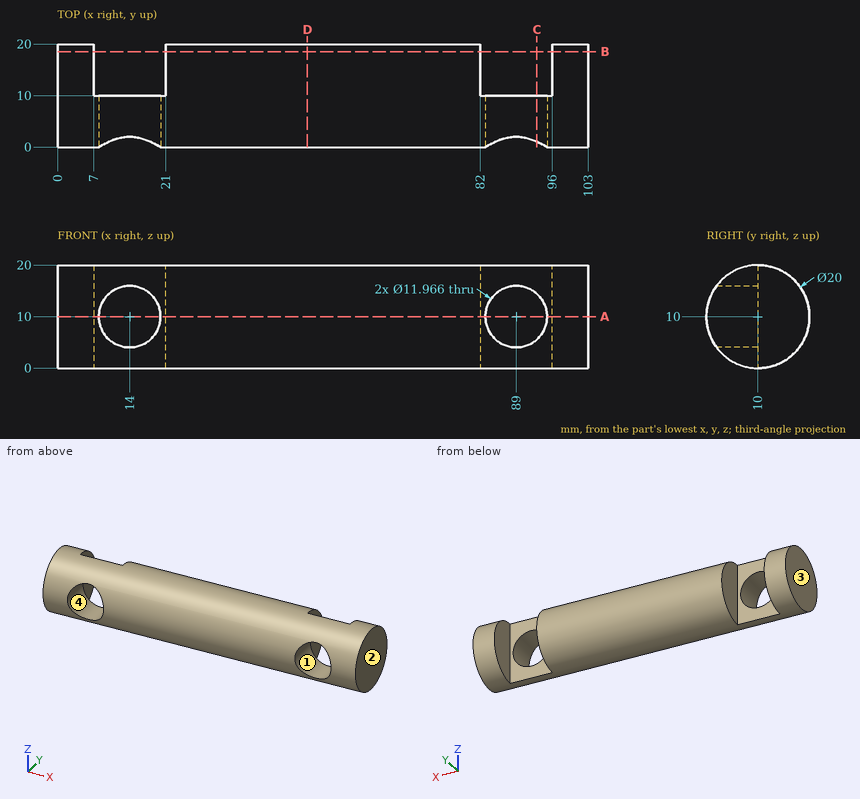
Geometry: see drawing. Coordinates: mm, zero at the bounding-box minimum. Round coordinates to 2 decimals unless told otherwise and drop trailing zeros. Loops run counter-clockwise (first coordinate to the right, second up) from the corner with the lowest first, then second, coordinate; pieces in that order, holes last.
(1) Section query A-A (z = 10). Output: boundary loops of the cut face in (x, y).
From the geometry:
outline: (0, 0) - (8.02, 0) - (8.02, 10) - (7, 10) - (7, 20) - (0, 20) - close; (19.98, 0) - (83.02, 0) - (83.02, 10) - (82, 10) - (82, 20) - (21, 20) - (21, 10) - (19.98, 10) - close; (94.98, 0) - (103, 0) - (103, 20) - (96, 20) - (96, 10) - (94.98, 10) - close
(2) Material intervals for probe 1 along X at (y, z) = (2.75, 10); probe 2 along X at (y, z) = (10.75, 17.5); probe 3 along Z at (x, y) = (72, 9.5), sorted ascending.
From the geometry:
probe 1: x = 0 to 8.02, 19.98 to 83.02, 94.98 to 103
probe 2: x = 0 to 7, 21 to 82, 96 to 103
probe 3: z = 0.01 to 19.99
(3) Section query C-C (x = 93). Output: boundary loops of the cut face in (y, z).
From the geometry:
outline: (1.04, 5.55) arc R10 ccw to (10, 0) - (10, 5.55) - close; (1.04, 14.45) - (10, 14.45) - (10, 20) arc R10 ccw to start
(4) Section query D-D (x = 48.5). Output: boundary loops of the cut face in (y, z), and give its area (3 significant figures).
From the geometry:
outline: circle Ø20 at (10, 10)
area: 314 mm2
(5) Contact query for flat-ended pins moving along their axis: pin 1 Ø10 at (x, y) = (56, 16) entering from +Z; pin 2 Ø3 at (x, z) = (84, 12) entering from -Y; pin 3 Ø3 at (x, z) = (46, 4.5) entering from +Y; pin 4 Ø11 at (x, z) = (14, 10) entering from -Y. Output: stop coordinate, or through.
From the geometry:
pin 1: stops at z = 19.95
pin 2: stops at y = 0.03
pin 3: stops at y = 19.17
pin 4: passes through
(6) Section query B-B (y = 18.5). Output: boundary loops of the cut face in (x, z).
From the geometry:
outline: (0, 4.73) - (7, 4.73) - (7, 15.27) - (0, 15.27) - close; (21, 4.73) - (82, 4.73) - (82, 15.27) - (21, 15.27) - close; (96, 4.73) - (103, 4.73) - (103, 15.27) - (96, 15.27) - close
(7) Pull-direction query (X, two-part tool) for the marked faces 1, 2, 3 and 4; classes: +X half, -X half, draft (parallel to the pull), parting line (faces both ways), or undercut.
From the geometry:
face 1: undercut
face 2: +X half
face 3: -X half
face 4: undercut
